Geometry: see drawing. Coordinates: mm, zero at the bounding-box minimum. Give positions to 0.01 mm unless a question says otherwise; leave off trailing zeros. Write each loop counter-clockwise with the first axis right and the second up, starting at its lowest first coordinate (ties: lowest second). Pieces come first, ordered by that corner, then holes. Notation, with made-up numbers: M -11,34.25 L 48,34.25 A15 ccw 48,45.25 Z; hole C 89,29.25 d11. An arc over 180 degrees is marked long. Use a Markdown table: item, result. Add a question column.
(1) Cut plane A-A (x = 35). Output: boundary loops of the cut face in (y, z), plus the area to 3 significant figures.
(2) Cut plane B-B (z = 0.65). Output: boundary loops of the cut face in (x, y), plus the area to 3 significant figures.
(3) Cut plane D-D (x = 4). Output: boundary loops of the cut face in (y, z), plus the area to 3 significant figures.
(4) Pin query (flat end, axial travel): pin 1 Ø1.8 at (x, y) = (20, 20.5) entering from +Z. Return the tip coordinate at first contact, or that it passes through.
(5) Material intervals for L1, parallel to Y at x = 35, z = 2.3; L2, parallel to Y at x = 5.5, z = 1.15; L3, parallel to X at y = 4.25, z = 0.45, sorted ascending.
(6) Cut plane C-C (y = 20.5). Output: boundary loops of the cut face in (x, z).
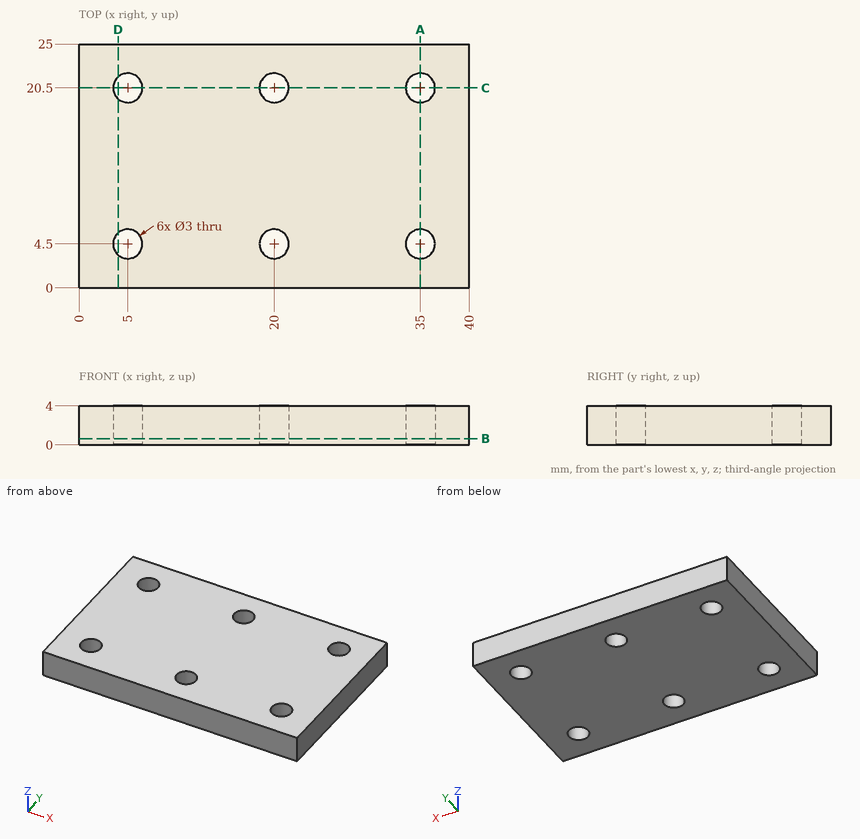
Answer list:
| question | item | result |
|---|---|---|
| 1 | outline | M 0,0 L 3,0 L 3,4 L 0,4 Z; M 6,0 L 19,0 L 19,4 L 6,4 Z; M 22,0 L 25,0 L 25,4 L 22,4 Z |
| 1 | area | 76.0 mm² |
| 2 | outline | M 0,0 L 40,0 L 40,25 L 0,25 Z; hole C 5,4.5 d3; hole C 5,20.5 d3; hole C 20,4.5 d3; hole C 20,20.5 d3; hole C 35,4.5 d3; hole C 35,20.5 d3 |
| 2 | area | 958 mm² |
| 3 | outline | M 0,0 L 3.38,0 L 3.38,4 L 0,4 Z; M 5.62,0 L 19.38,0 L 19.38,4 L 5.62,4 Z; M 21.62,0 L 25,0 L 25,4 L 21.62,4 Z |
| 3 | area | 82.1 mm² |
| 4 | pin 1 | through |
| 5 | L1 | 0 to 3, 6 to 19, 22 to 25 |
| 5 | L2 | 0 to 3.09, 5.91 to 19.09, 21.91 to 25 |
| 5 | L3 | 0 to 3.52, 6.48 to 18.52, 21.48 to 33.52, 36.48 to 40 |
| 6 | outline | M 0,0 L 3.5,0 L 3.5,4 L 0,4 Z; M 6.5,0 L 18.5,0 L 18.5,4 L 6.5,4 Z; M 21.5,0 L 33.5,0 L 33.5,4 L 21.5,4 Z; M 36.5,0 L 40,0 L 40,4 L 36.5,4 Z |
